Model file for the job. Use its own axes, mm. A direction names the side the tool comes from. Round coordinates to 2 decimals unless told otherwise and drop trailing zeros. Loops run counter-clockwise (first coordinate to the right, second up) from the corner with the lowest first, then second, coordinate; pieces in that order, holes last. Notation, with made-up numbers: (50.25, 6.5) -> (55.25, 6.5) arc R16 ccw to (55.25, 25.5) -> close; hole circle Ø8 at (-31.5, 8). An arc over 180 degrees is marked (long way). Use a Markdown table: item, result.
Autodesk Inventor part; units mm, degrees
ref_plane "CP_PLATE_XY" through (0, 15.5, 0) normal (0, 0, 1) x (1, 0, 0)
ref_plane "CP_PLATE_YZ" through (0, 15.5, 0) normal (1, 0, 0) x (0, 1, 0)
ref_plane "CP_PLATE_ZX" through (0, 15.5, 0) normal (0, 1, 0) x (0, 0, 1)
sketch "Sketch_1" plane through (0, 0, 0) normal (0, 0, 1) x (1, 0, 0)
  line L0 (-7.5, 24) -> (-7.5, 0)
  line L1 (-7.5, 0) -> (7.5, 0)
  line L2 (7.5, 0) -> (7.5, 24)
  line L3 (7.5, 24) -> (-7.5, 24)
extrude "Extrusion1" add sketch "Sketch_1" against normal blind 7
sketch "Sketch_3" plane through (0, 0, 0) normal (0, 0, 1) x (1, 0, 0)
  arc A0 (-0.5, 18.458) -> (0.5, 18.458) centre (0, 15.5) ccw
  line L0 (0.5, 18.458) -> (0.5, 24)
  line L1 (0.5, 24) -> (-0.5, 24)
  line L2 (-0.5, 24) -> (-0.5, 18.458)
extrude "Extrusion2" cut sketch "Sketch_3" against normal blind 7
sketch "Sketch3" plane through (7.5, 0, 0) normal (1, 0, 0) x (0, 0, -1)
  point P0 (3.5, 20.5)
hole "Hole1" at (7.5, 20.5, -3.5) direction (-1, 0, 0) diameter 3.4 depth 7.5 counterbore diameter 5.9 counterbore depth 3.5
sketch "Sketch4" plane through (-7.5, 0, 0) normal (-1, 0, 0) x (0, 0, 1)
  point P0 (-3.5, 20.5)
hole "Hole2" at (-7.5, 20.5, -3.5) direction (1, 0, 0) diameter 2.459 depth 7
sketch "Sketch_6" plane through (0, 0, 0) normal (1, 0, 0) x (0, 1, 0)
  line L0 (2.2, -65) -> (2.2, 0)
  line L1 (2.2, 0) -> (3.7, 0)
  line L2 (3.7, 0) -> (3.7, -64.6)
  line L3 (3.7, -64.6) -> (3.3, -65)
  line L4 (3.3, -65) -> (2.2, -65)
  line L5 (2.2, -65) -> (2.2, 0)
revolve "Revolution1" add sketch "Sketch_6" angle 360 about axis through (0, 2.2, -65) along (0, 0, -1)
ref_plane "CP_PLATE_XY" through (0, 15.5, 0) normal (0, 0, 1) x (1, 0, 0)
ref_plane "CP_PLATE_YZ" through (0, 15.5, 0) normal (1, 0, 0) x (0, 1, 0)
ref_plane "CP_PLATE_ZX" through (0, 15.5, 0) normal (0, 1, 0) x (0, 0, 1)
ref_plane "CP_SCREW_XY" through (4, 20.5, -3.5) normal (1, 0, 0) x (0, 0, -1)
ref_plane "CP_SCREW_YZ" through (4, 20.5, -3.5) normal (0, 0, -1) x (0, 1, 0)
ref_plane "CP_SCREW_ZX" through (4, 20.5, -3.5) normal (0, 1, 0) x (1, 0, 0)
properties part number "4186566 DPDM 16-50---(p)"
Q1. Tool access for faces 4 (the face through (0.5, 22.4, -3.5)), 5 (the face through (5.726, 18.506, -1.326)), 6 (the face through (-0.1, 12.5, -3.5)), 7 (the face through (-0.575, 3.586, -36.203)): list every direction of +Z, -Z, +X, -X, +Y, -Y with a clear straight run to the whole face (end or side of a thin tool).
Results list:
| item | result |
|---|---|
| face 4 | +Z, -Z, +Y |
| face 5 | +X |
| face 6 | +Z, -Z |
| face 7 | -Z |
Q2. Pull direction Y, two halves, no side cores. Call faces 1 (the face through (-7.5, 12, -3)), 2 (the face through (-3.95, 21.7, -3.77)), 3 (the face through (-4, 24, -3)): released by +Y, released by -Y, zero draft, split by the parting line, or undercut.
Results list:
| item | result |
|---|---|
| face 1 | zero draft |
| face 2 | undercut |
| face 3 | released by +Y |
Q3. Band-saw the part on D-D, the plane y = 2.2. Give the cut face in (x, z).
Results list:
| item | result |
|---|---|
| outline | (-7.5, -7) -> (-1.5, -7) -> (-1.5, -64.6) -> (-1.1, -65) -> (1.1, -65) -> (1.5, -64.6) -> (1.5, -7) -> (7.5, -7) -> (7.5, 0) -> (-7.5, 0) -> close |
Q4. Band-saw the part on B-B, the plane z = -3.5. Give the cut face in (x, y), plus the area to 3 significant figures.
Results list:
| item | result |
|---|---|
| outline | (-7.5, 0) -> (7.5, 0) -> (7.5, 17.55) -> (4, 17.55) -> (4, 18.8) -> (0.5, 18.8) -> (0.5, 18.46) arc R3 cw (long way) to (-0.5, 18.46) -> (-0.5, 19.27) -> (-7.5, 19.27) -> close; (-7.5, 21.73) -> (-0.5, 21.73) -> (-0.5, 24) -> (-7.5, 24) -> close; (0.5, 22.2) -> (4, 22.2) -> (4, 23.45) -> (7.5, 23.45) -> (7.5, 24) -> (0.5, 24) -> close |
| area | 276 mm² |
Q5. Band-saw the part on C-C, the plane y = 15.5. Give the cut face in (x, z), plus the area to 3 significant figures.
Results list:
| item | result |
|---|---|
| outline | (-7.5, -7) -> (-3, -7) -> (-3, 0) -> (-7.5, 0) -> close; (3, -7) -> (7.5, -7) -> (7.5, 0) -> (3, 0) -> close |
| area | 63.0 mm² |
Q6. Band-saw the part on A-A, the plane y = 20.5. Give the cut face in (x, z), plus the area to 3 significant figures.
Results list:
| item | result |
|---|---|
| outline | (-7.5, -7) -> (-0.5, -7) -> (-0.5, -4.73) -> (-7.5, -4.73) -> close; (-7.5, -2.27) -> (-0.5, -2.27) -> (-0.5, 0) -> (-7.5, 0) -> close; (0.5, -7) -> (7.5, -7) -> (7.5, -6.45) -> (4, -6.45) -> (4, -5.2) -> (0.5, -5.2) -> close; (0.5, -1.8) -> (4, -1.8) -> (4, -0.55) -> (7.5, -0.55) -> (7.5, 0) -> (0.5, 0) -> close |
| area | 48.2 mm² |
Q7. Drill centre lines: L1, parallel to Z at x = -5.25, y = 20.5; L2, parallel to Y at x = 5.65, z = -3.5; L3, parallel to Z at x = 5.05, y = 20.5. Where is each one in solid material? Low to high. Write a range as from..to.
Results list:
| item | result |
|---|---|
| L1 | z = -7..-4.73, -2.27..0 |
| L2 | y = 0..17.55, 23.45..24 |
| L3 | z = -7..-6.45, -0.55..0 |
Q8. Flat gauge pins, fed straight in: pin 1 (3.5 mm diameter, centred on y = 20.5, z = -3.5, fed in from +X); pin 2 (1.5 mm diameter, centred on x = 4.5, y = 13.5, fed in from -Z). Where does each tip first touch, or does it go through?
Results list:
| item | result |
|---|---|
| pin 1 | stops at x = 4 |
| pin 2 | stops at z = -7 |
